```python
from build123d import *

# Parameters (mm, degrees)
F0_W     = 1000
F0_H     = 120.975018
F2_DEPTH = 1000
F1_W     = 4.91416
F1_H     = 44.66103
F3_DEPTH = 1000


with BuildPart() as f2:
    # F0 (on Front) → F2 (new body)
    with BuildSketch(Plane.XZ):
        with Locations((292.73814, 60.487509)):
            Rectangle(F0_W, F0_H)
    extrude(amount=F2_DEPTH)

    # F1 (on Front) → F3 (cut)
    with BuildSketch(Plane.XZ):
        with Locations((2.45708, 22.330515)):
            Rectangle(F1_W, F1_H)
        with BuildLine():
            Line((0, 44.66103), (4.91416, 44.66103))
            ThreePointArc((4.91416, 44.66103), (2.45708, 47.11811), (0, 44.66103))
        make_face()
    extrude(amount=F3_DEPTH, mode=Mode.SUBTRACT)


solid = f2.part
```
Could you check a few things on this model? Use its own coordinates, in mm. A direction names the side the tool comes from. Round coordinates to 2 decimals unless told otherwise and drop trailing zeros. One line per question, with ' | ' between items.
Q1. If I drill on line 1 (X direction, y = -627.5, z = 17), over which ranges is the centre line in solid material (lowest first)? Write a range as from..to.
Computed values:
line 1: -207.26..0, 4.91..792.74
Q2. We'd pull the mould along X, two halves only. Please class faces 1 (the face through (4.914, -493, 22)), 2 (the face through (286, -493, 120.975)), 3 (the face through (-207.262, -493, 60)): released by +X, released by -X, zero draft, split by the parting line, or undercut.
Computed values:
face 1: undercut | face 2: zero draft | face 3: released by -X
Q3. Which directions (+Z, -Z, +X, -X, +Y, -Y) give clear straight access to the entire face, cutting with the end or side of a thin tool? Please do faces 4 (the face through (0, -493, 22)), 5 (the face through (-105, -493, 0)).
Computed values:
face 4: -Z, +Y, -Y | face 5: -Z, +X, -X, +Y, -Y
